Could you check a few things on this model? Use its own coordinates, in mm. Face numbers are marked on the shaded views. Round coordinates to 2 decimals unless told otherwise and drop trailing zeros. One line per item, written item: value.
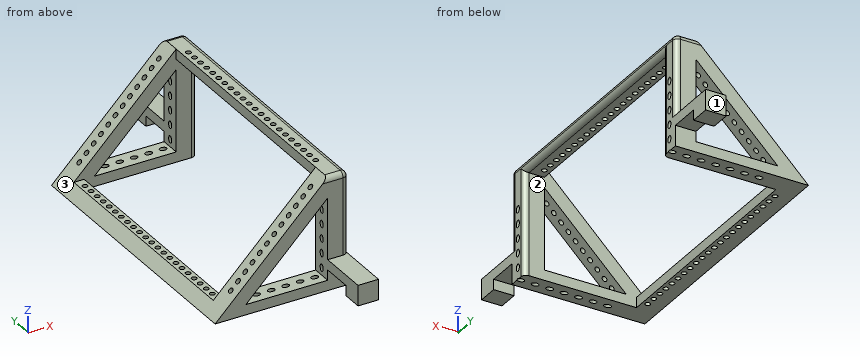
```python
from build123d import *

# Parameters (mm, degrees)
F1_DEPTH  = 10
F3_DEPTH  = 20
F4_W      = 10
F4_H      = 10
F5_DEPTH  = 20
F6_W      = 10
F6_H      = 10
F7_DEPTH  = 20
F8_W      = 10
F8_H      = 10
F9_DEPTH  = 20
F11_DEPTH = 10
F13_DEPTH = 20
F14_DEPTH = 20
F15_DEPTH = 10
F17_DEPTH = 20
F18_DEPTH = 10
F20_R     = 4.99999
F22_D     = 5
F23_DEPTH = 250
F25_D     = 5
F27_D     = 5


# Not quite as in the source:
# - a fillet or chamfer is up to 0.001 mm smaller than in the source, because OpenCascade refuses the exact size
# - a pattern or mirror of a feature is missing from the dataset's text; its kind, count and spacing are read off the source's solid


with BuildPart() as f1:
    # F0 (on Right) → F1 (new body)
    with BuildSketch(Plane.YZ):
        Polygon((0, -100), (0, 0), (250, 0), (250, -100), (260, -100), (260, 10), (-10, 10), (-10, -100), align=None)
    extrude(amount=F1_DEPTH)

    # F2 (on face) → F3 (join)
    with BuildSketch(Plane.YZ.offset(10)):
        Polygon((-40, -80), (-10, -80), (-10, -70), (-60, -70), (-60, -90), (-40, -90), align=None)
        Polygon((310, -70), (260, -70), (260, -80), (290, -80), (290, -90), (310, -90), align=None)
    extrude(amount=-F3_DEPTH)

    # F4 (on face) → F5 (join)
    with BuildSketch(Plane.YZ.offset(10)):
        with Locations((-5, -75)):
            Rectangle(F4_W, F4_H)
        with Locations((255, -75)):
            Rectangle(F4_W, F4_H)
    extrude(amount=-F5_DEPTH)

    # F6 (on face) → F7 (join)
    with BuildSketch(Plane(origin=(0, 0, -80), x_dir=(1, 0, 0), z_dir=(0, 0, -1))):
        with Locations((-5, -255)):
            Rectangle(F6_W, F6_H)
    extrude(amount=F7_DEPTH)

    # F8 (on face) → F9 (join)
    with BuildSketch(Plane(origin=(0, 0, -80), x_dir=(1, 0, 0), z_dir=(0, 0, -1))):
        with Locations((-5, 5)):
            Rectangle(F8_W, F8_H)
    extrude(amount=F9_DEPTH)

    # F10 (on face) → F11 (join)
    with BuildSketch(Plane(origin=(0, 0, 0), x_dir=(0, -1, 0), z_dir=(-1, 0, 0))):
        Polygon((10, 10), (-260, 10), (-260, -70), (-250, -70), (-250, 0), (0, 0), (0, -70), (10, -70), align=None)
    extrude(amount=F11_DEPTH)

    # F12 (on face) → F13 (join)
    with BuildSketch(Plane.XZ.offset(10)):
        Polygon((-10, 0), (-10, 10), (-110, -90), (-100, -90), align=None)
        Polygon((-10, -90), (-90, -90), (-100, -100), (-10, -100), align=None)
        Polygon((-100, -90), (-110, -90), (-110, -100), align=None)
        Polygon((-110, -100), (-110, -90), (-120, -100), align=None)
    extrude(amount=-F13_DEPTH)

    # F12 (on face) → F14 (join)
    with BuildSketch(Plane.XZ.offset(10)):
        Polygon((10, 10), (-10, 10), (-10, 0), (-10, -10), (-10, -70), (10, -70), align=None)
        Polygon((-90, -90), (-100, -90), (-110, -100), (-100, -100), align=None)
    extrude(amount=-F14_DEPTH)

    # F15 (add): a face of the model
    f15_faces = [f1.faces().sort_by_distance(p)[0] for p in [
        (0, 0, -85),
    ]]
    extrude(f15_faces, amount=F15_DEPTH)

    # F16 (on face) → F17 (join)
    with BuildSketch(Plane(origin=(0, 260, 0), x_dir=(-1, 0, 0), z_dir=(0, 1, 0))):
        Polygon((110, -90), (10, 10), (10, -10), (90, -90), align=None)
        Polygon((120, -100), (110, -90), (90, -90), (10, -90), (10, -100), align=None)
    f17 = extrude(amount=-F17_DEPTH)

    # F17_copies: F17 across plane
    add(f17.mirror(Plane(origin=(0, 125, 0), x_dir=(0, 0, -1), z_dir=(0, -1, 0))))

    # F18 (add): a face of the model
    f18_faces = [f1.faces().sort_by_distance(p)[0] for p in [
        (0, 250, -50),
    ]]
    extrude(f18_faces, amount=F18_DEPTH)

    # F20 (radius 5 in the source; OpenCascade refuses exactly that, so slightly less here)
    f20_edges = [f1.edges().sort_by_distance(p)[0] for p in [
        (10, 125, 10),
        (10, 125, 0),
        (10, 10, -50),
        (10, 240, -50),
        (10, -10, -30),
        (10, 260, -30),
        (0, 260, 10),
        (0, -10, 10),
    ]]
    fillet(f20_edges, radius=F20_R)

    # F22 (through all)
    with Locations(Plane.XY.offset(10)):
        with Locations((-4, 20), (-4, 30), (-4, 40), (-4, 50), (-4, 60), (-4, 70), (-4, 80), (-4, 90), (-4, 100), (-4, 110), (-4, 120), (-4, 130), (-4, 140), (-4, 150), (-4, 140), (-4, 160), (-4, 170), (-4, 180), (-4, 200), (-4, 210), (-4, 220), (-4, 230), (-4, 190)):
            Hole(F22_D / 2)

    # F19 (on face) → F23 (join)
    with BuildSketch(Plane.XZ.offset(-240)):
        Polygon((-100, -100), (-100, -90), (-110, -90), (-120, -100), align=None)
    extrude(amount=F23_DEPTH)

    # F25 (through all)
    with Locations(Plane.XY.offset(-90)):
        with Locations((-105, 20), (-105, 30), (-105, 40), (-105, 50), (-105, 60), (-105, 70), (-105, 80), (-105, 90), (-105, 100), (-105, 110), (-105, 120), (-105, 130), (-105, 140), (-105, 150), (-105, 160), (-105, 170), (-105, 180), (-105, 190), (-105, 200), (-105, 210), (-105, 220), (-105, 230)):
            Hole(F25_D / 2)

    # F27 (through all)
    with Locations(Plane(origin=(-10, 0, 10), x_dir=(0, -1, 0), z_dir=(-0.7071067812, 0, 0.7071067812))):
        with Locations((0, -15.563491861), (0, -25.563491861), (0, -35.563491861), (0, -45.563491861), (0, -55.563491861), (0, -65.563491861), (0, -75.563491861), (0, -85.563491861), (0, -95.563491861), (0, -105.563491861), (0, -115.563491861), (0, -125.563491861), (-250, -15.563491861), (-250, -25.563491861), (-250, -35.563491861), (-250, -45.563491861), (-250, -55.563491861), (-250, -65.563491861), (-250, -75.563491861), (-250, -85.563491861), (-250, -95.563491861), (-250, -105.563491861), (-250, -115.563491861), (-250, -125.563491861)):
            Hole(F27_D / 2)


solid = f1.part
```
(1) For pin 1 Ø6 at (x, y) = (-4, 230) entering from -Z; pin 2 Ø6 at (x, y) = (-2.5, -27) entering from -Z; pin 3 Ø6.5 at (x, y) = (-105, 230) entering from +Z, each with a flat end and sliding along its axis, tell me the tip position at first contact or that it passes through.
Results below:
pin 1: stops at z = 0
pin 2: stops at z = -80
pin 3: stops at z = -90
(2) Please list where these lines run through material, in increasing order: L1, parallel to Y at x = -90, z = -75; L2, parallel to Y at x = -96, z = -77; L3, parallel to Z at x = -100, y = 244.5.
Results below:
L1: y = -10 to -2.24, 2.24 to 10, 240 to 247.76, 252.24 to 260
L2: y = -10 to 10, 240 to 260
L3: z = -100 to -80
(3) We'd pull the mould along Y, two halves only. Please class the marked faces 1, 2 and 3: +Y half, -Y half, draft (parallel to the pull), parting line (faces both ways), or undercut.
Results below:
face 1: +Y half
face 2: undercut
face 3: draft
